The model under review builds one solid part; all positions refer to its coordinate system, in mm. Face numbers are marked on the shaded views. A direction names the side the tool comes from. Round coordinates to 2 decimals unless told otherwise and drop trailing zeros. Write each loop counter-clockwise with the first axis right and the second up, starting at its lowest first coordinate (ties: lowest second). Pieces come first, ordered by that corner, then holes. Notation, with made-up numbers: (-29, -30.5) - (4, -30.5) arc R31 ccw to (4, 6.5) - close; hole circle Ø11 at (44.5, 56.5). An arc over 180 degrees is marked (long way). Use one line per item in the form item = value.
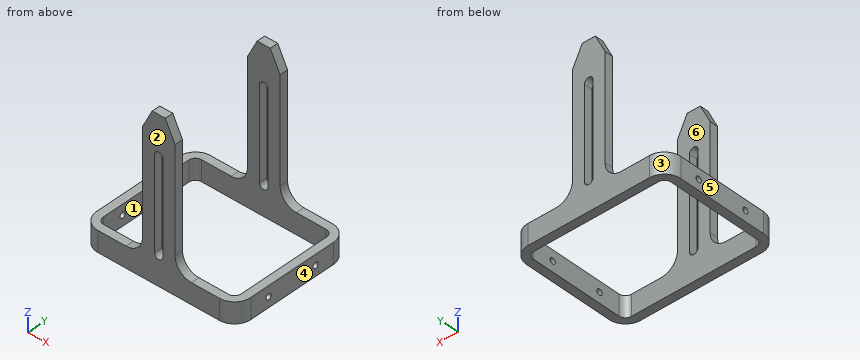
from build123d import *

# Parameters (mm, degrees)
SKETCH1_W             = 59.944
SKETCH1_H             = 47.752
SKETCH1_W_2           = 53.594
SKETCH1_H_2           = 41.402
BOSS_EXTRUDE1_DEPTH   = 8.001
BOSS_EXTRUDE2_DEPTH   = 3.175
CUT_EXTRUDE1_DEPTH    = 3.302
F_4_40_TAPPED_HOLE1_D = 2.2606
FILLET1_R             = 6.35
FILLET2_R             = 2.54
FILLET3_R             = 6.35


with BuildPart() as part:
    # Sketch1 → Boss-Extrude1 (new body)
    with BuildSketch(Plane.XY):
        Rectangle(SKETCH1_W, SKETCH1_H)
        Rectangle(SKETCH1_W_2, SKETCH1_H_2, mode=Mode.SUBTRACT)
    extrude(amount=BOSS_EXTRUDE1_DEPTH)

    # Sketch2 → Boss-Extrude2 (add)
    with BuildSketch(Plane(origin=(0, 23.876, 0), x_dir=(1, 0, 0), z_dir=(0, 1, 0))):
        Polygon((-6.35, -8.001), (-6.35, -54.61), (-2.54, -62.23), (2.54, -62.23), (6.35, -54.61), (6.35, -8.001), align=None)
    boss_extrude2 = extrude(amount=-BOSS_EXTRUDE2_DEPTH)

    # Sketch3 → Cut-Extrude1 (cut)
    with BuildSketch(Plane(origin=(0, 23.876, 0), x_dir=(1, 0, 0), z_dir=(0, 1, 0))):
        with BuildLine():
            Line((-1.651, -46.99), (-1.651, -11.43))
            ThreePointArc((-1.651, -11.43), (0, -9.779), (1.651, -11.43))
            Line((1.651, -11.43), (1.651, -46.99))
            ThreePointArc((1.651, -46.99), (0, -48.641), (-1.651, -46.99))
        make_face()
    cut_extrude1 = extrude(amount=-CUT_EXTRUDE1_DEPTH, mode=Mode.SUBTRACT)

    # Mirror1: Boss-Extrude2, Cut-Extrude1 across plane
    add(boss_extrude2.mirror(Plane.ZX))
    add(cut_extrude1.mirror(Plane.ZX), mode=Mode.SUBTRACT)

    # #4-40 Tapped Hole1 (through all)
    with Locations(Plane.ZY.offset(29.972)):
        with Locations((4.0005, 9.9441), (4.0005, -9.9441)):
            Hole(F_4_40_TAPPED_HOLE1_D / 2)

    # Fillet1
    fillet1_edges = [part.edges().sort_by_distance(p)[0] for p in [
        (29.972, -23.876, 4.0005),
        (-29.972, -23.876, 4.0005),
        (-29.972, 23.876, 4.0005),
        (29.972, 23.876, 4.0005),
    ]]
    fillet(fillet1_edges, radius=FILLET1_R)

    # Fillet2
    fillet2_edges = [part.edges().sort_by_distance(p)[0] for p in [
        (26.797, -20.701, 4.0005),
        (26.797, 20.701, 4.0005),
        (-26.797, 20.701, 4.0005),
        (-26.797, -20.701, 4.0005),
    ]]
    fillet(fillet2_edges, radius=FILLET2_R)

    # Fillet3
    fillet3_edges = [part.edges().sort_by_distance(p)[0] for p in [
        (-6.35, 22.2885, 8.001),
        (6.35, 22.2885, 8.001),
        (-6.35, -22.2885, 8.001),
        (6.35, -22.2885, 8.001),
    ]]
    fillet(fillet3_edges, radius=FILLET3_R)


solid = part.part
(1) To check wall thickness, follow L1, parallel to Y at x = 18.5, z = 7; L2, parallel to X at y = -13.5, z = 6; L3, parallel to X at y = -21, z = 15. State the ranges of each line that lie inside material, in increasing order.
Geometry results:
L1 = -23.88 to -20.7, 20.7 to 23.88
L2 = -29.97 to -26.8, 26.8 to 29.97
L3 = -6.35 to -1.65, 1.65 to 6.35
(2) Add section A-A on x = 3.5. Write out the cut boundary in (y, z).
Geometry results:
outline = (-23.88, 0) - (-20.7, 0) - (-20.7, 60.31) - (-23.88, 60.31) - close; (20.7, 0) - (23.88, 0) - (23.88, 60.31) - (20.7, 60.31) - close
(3) Add section C-C on z = 37.5. Write out the cut boundary in (x, y).
Geometry results:
outline = (-6.35, -23.88) - (-1.65, -23.88) - (-1.65, -20.7) - (-6.35, -20.7) - close; (-6.35, 20.7) - (-1.65, 20.7) - (-1.65, 23.88) - (-6.35, 23.88) - close; (1.65, -23.88) - (6.35, -23.88) - (6.35, -20.7) - (1.65, -20.7) - close; (1.65, 20.7) - (6.35, 20.7) - (6.35, 23.88) - (1.65, 23.88) - close
(4) Insertion check: P1, Ø1, axis at y = -21.5, z = 34.5, coming from the +X side; P2, Ø1, axis at y = 22, z = 30, coming from the -X side; P3, Ø8.5, axis at x = -21, y = -10, coming from the +Z side; P4, Ø14, axis at x = 22, y = 3, coming from the +Z side. Each pin has a flat end and moves straight along its axis. Give the tip position at first contact, or say it passes through.
Geometry results:
P1 = 6.35
P2 = -6.35
P3 = through
P4 = 8
(5) Machinability: for the marked faces 5 and 6, which of the approach directions +Z, -Z, +X, -X, +Y, -Y give a long, thin tool a straight path to every point of the face, cutting with its end or side? Answer none if there is none.
Geometry results:
face_5 = +Z, -Z, -X, +Y, -Y
face_6 = +Z, -Z
(6) The part is to be moulded in two halves that separate along Y. For the marked faces 1, 2, 3 and 4, say which applies: +Y half, -Y half, draft (parallel to the pull), parting line (faces both ways), or undercut.
Geometry results:
face_1 = undercut
face_2 = -Y half
face_3 = +Y half
face_4 = draft
(7) Add section B-B on y = 6. Write out the cut boundary in (x, z), then the cut area to 3 significant figures.
Geometry results:
outline = (-29.97, 0) - (-26.8, 0) - (-26.8, 8) - (-29.97, 8) - close; (26.8, 0) - (29.97, 0) - (29.97, 8) - (26.8, 8) - close
area = 50.8 mm2
